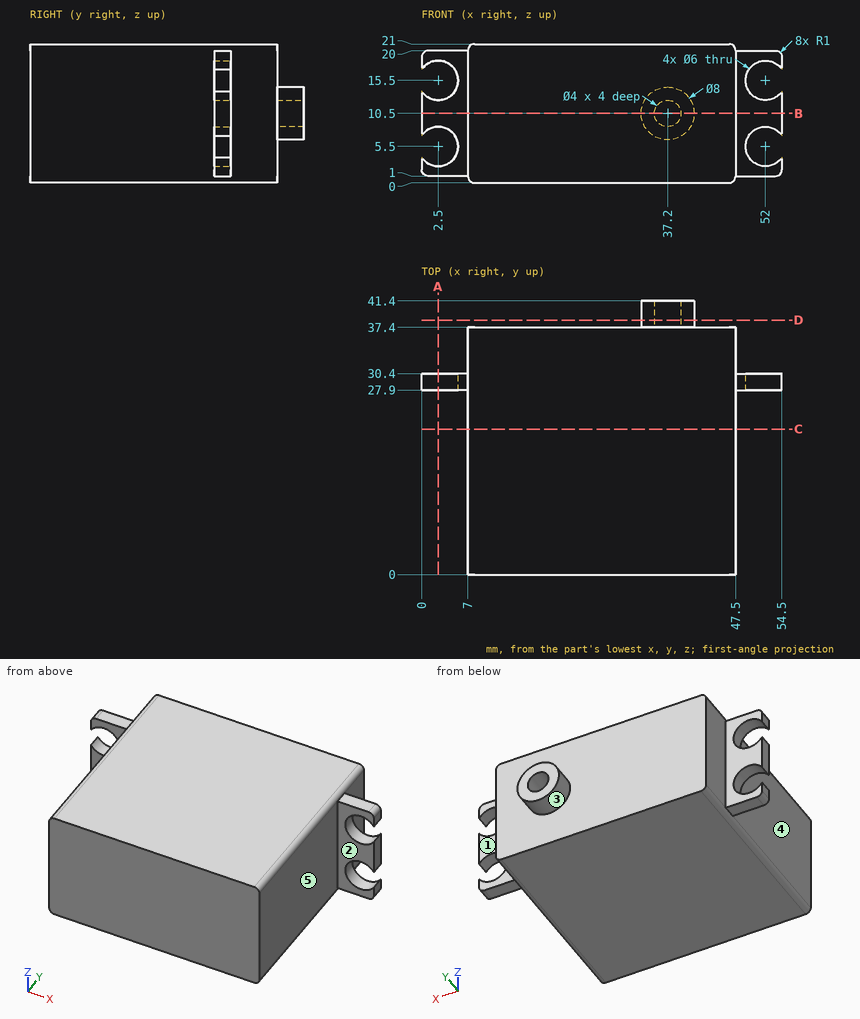
Can you work these out from the drawing? Everything is in mm from the part's minimum corner. A direction names the side the tool comes from. Round coordinates to 2 decimals unless told otherwise and drop trailing zeros. Loops run counter-clockwise (first coordinate to the right, second up) from the corner with the lowest first, then second, coordinate; pieces in that order, holes last. Notation, with made-up numbers: (21, 60) - (72, 60) arc R34 cw to (72, 98) - close; hole circle Ø2 at (72.25, 36). An arc over 180 degrees is marked (long way). Answer in a Markdown table with one row per item. Add a question column.
(1) If we section it at B-B (z = 10.5): Please give me the cut outline in (x, y).
(2) I'm going to push flat-ended pins straight in: pin 1 (12 mm diameter, centred on y = 31, z = 14, fed in from -X); pin 2 (1.2 mm diameter, centred on x = 36.5, z = 10.5, fed in from +Y); pin 3 (5.5 mm diameter, centred on x = 4, z = 6, fed in from -Y); pin 4 (3.5 mm diameter, centred on x = 51, z = 10, fed in from +Y). Where does each tip first touch, or does it pass through?
(3) I need wall thicknesses on line 1 along Z through (x, y) = (2.5, 29.2); line 2 along X through (y, z) = (39.95, 10.5); line 3 along Y through (x, z) = (16, 11.25). Which ranges of each line are inside material? Lowest first, please.
(4) If we section it at A-A (x = 2.5): Please give me the cut outline in (y, z), plus the area to 3 significant figures.
(5) If we section it at C-C (y = 22): Please give me the cut outline in (x, z).
(6) For the marked faces 1, 2, 3, 4 and 5, which set-ups out of +Z, -Z, +X, -X, +Y, -Y let a thin tool reach every point of the face, with its end or its side?
(7) If we section it at D-D (y = 38.5): Please give me the cut outline in (x, z), plus the area to 3 significant figures.
Model answer:
| question | item | result |
|---|---|---|
| 1 | outline | (0, 27.9) - (7, 27.9) - (7, 0) - (47.5, 0) - (47.5, 27.9) - (54.5, 27.9) - (54.5, 30.4) - (47.5, 30.4) - (47.5, 37.4) - (41.2, 37.4) - (41.2, 41.4) - (39.2, 41.4) - (39.2, 37.4) - (35.2, 37.4) - (35.2, 41.4) - (33.2, 41.4) - (33.2, 37.4) - (7, 37.4) - (7, 30.4) - (0, 30.4) - close |
| 2 | pin 1 | stops at x = 0 |
| 2 | pin 2 | stops at y = 37.4 |
| 2 | pin 3 | stops at y = 27.9 |
| 2 | pin 4 | stops at y = 30.4 |
| 3 | line 1 | z = 1 to 2.5, 8.5 to 12.5, 18.5 to 20 |
| 3 | line 2 | x = 33.2 to 35.2, 39.2 to 41.2 |
| 3 | line 3 | y = 0 to 37.4 |
| 4 | outline | (27.9, 1) - (30.4, 1) - (30.4, 2.5) - (27.9, 2.5) - close; (27.9, 8.5) - (30.4, 8.5) - (30.4, 12.5) - (27.9, 12.5) - close; (27.9, 18.5) - (30.4, 18.5) - (30.4, 20) - (27.9, 20) - close |
| 4 | area | 17.5 mm² |
| 5 | outline | (7, 1) arc R1 ccw to (8, 0) - (46.5, 0) arc R1 ccw to (47.5, 1) - (47.5, 20) arc R1 ccw to (46.5, 21) - (8, 21) arc R1 ccw to (7, 20) - close |
| 6 | face 1 | +Z, -Z, +X, +Y |
| 6 | face 2 | +Z, -Z, +X, -Y |
| 6 | face 3 | +Y |
| 6 | face 4 | +Z, -Z, -X, -Y |
| 6 | face 5 | +Z, -Z, +X, -Y |
| 7 | outline | circle Ø8 at (37.2, 10.5); hole circle Ø4 at (37.2, 10.5) |
| 7 | area | 37.7 mm² |
